```python
from build123d import *

# Parameters (mm, degrees)
SKETCH1_W                      = 40.11
SKETCH1_H                      = 20
BOSS_EXTRUDE1_DEPTH            = 12
SKETCH2_W                      = 35
SKETCH2_H                      = 17
BOSS_EXTRUDE2_DEPTH            = 6
SHELL1_START                   = 3.155
SHELL1_DEPTH                   = 33.8
SHELL1_START_2                 = 0.6
SHELL1_2_OUTLINE_W             = 18.8
SHELL1_2_OUTLINE_H             = 22.8
SHELL1_2_DEPTH                 = 38.91
SHELL1_START_3                 = -3.9
SHELL1_3_OUTLINE_R             = 0.1
SHELL1_3_DEPTH                 = 4.5
CUT_EXTRUDE1_REACH             = 48.398
SKETCH4_W                      = 30.63
SKETCH4_H                      = 5.52
CUT_EXTRUDE1_DIRECTION_2_REACH = 48.398
BOSS_EXTRUDE3_START            = 9.13
SKETCH5_W                      = 10.98
SKETCH5_H                      = 24.92
BOSS_EXTRUDE3_DEPTH            = 1.74
FILLET1_R                      = 2


# Read off the part's stored shape, not the designer's step: Shell1
with BuildPart() as part:
    # Sketch1 → Boss-Extrude1 (new, symmetric)
    with BuildSketch(Plane.XY):
        with Locations((20.055, 10)):
            Rectangle(SKETCH1_W, SKETCH1_H)
    extrude(amount=BOSS_EXTRUDE1_DEPTH, both=True)

    # Sketch2 → Boss-Extrude2 (add, symmetric)
    with BuildSketch(Plane.XY):
        with Locations((20.055, -8.5)):
            Rectangle(SKETCH2_W, SKETCH2_H)
    extrude(amount=BOSS_EXTRUDE2_DEPTH, both=True)

    # Sketch3 → Revolve1 (revolve)
    with BuildSketch(Plane.XY, mode=Mode.PRIVATE) as revolve1_sk:
        with BuildLine():
            Line((0, 0), (-3.5, 0))
            Line((-3.5, 0), (-3.5, -0.45))
            Line((-3.5, -0.45), (-4, -0.45))
            ThreePointArc((-4, -0.45), (-4.353553391, -0.303553391), (-4.5, 0.05))
            Line((-4.5, 0.05), (-4.5, 0.7))
            Line((-4.5, 0.7), (0, 0.7))
            Line((0, 0.7), (0, 0))
        make_face()
    revolve(revolve1_sk.sketch.rotate(Axis((0, 0.7, 0), (-1, 0, 0)), 180), axis=Axis((0, 0.7, 0), (-1, 0, 0)))

    # Shell1 outline → Shell1 (cut)
    with BuildSketch(Plane.YZ.offset(SHELL1_START)):
        Polygon((0.6, -5.4), (0.6, -11.4), (19.4, -11.4), (19.4, 11.4), (0.6, 11.4), (0.6, 5.4), (-17, 5.4), (-17, -5.4), align=None)
    extrude(amount=SHELL1_DEPTH, mode=Mode.SUBTRACT)

    # Shell1 2 outline → Shell1 2 (cut)
    with BuildSketch(Plane.YZ.offset(SHELL1_START_2)):
        with Locations((10, 0)):
            Rectangle(SHELL1_2_OUTLINE_W, SHELL1_2_OUTLINE_H)
    extrude(amount=SHELL1_2_DEPTH, mode=Mode.SUBTRACT)

    # Shell1 3 outline → Shell1 3 (cut)
    with BuildSketch(Plane.YZ.offset(SHELL1_START_3)):
        with Locations((0.7, 0)):
            Circle(SHELL1_3_OUTLINE_R)
    extrude(amount=SHELL1_3_DEPTH, mode=Mode.SUBTRACT)

    # Sketch4 → Cut-Extrude1 (cut, up to next)
    with BuildSketch(Plane.XY, mode=Mode.PRIVATE) as cut_extrude1_sk1:
        with Locations((20.055, -2.76)):
            Rectangle(SKETCH4_W, SKETCH4_H)
    cut_extrude1_tool1 = extrude(cut_extrude1_sk1.sketch, amount=-CUT_EXTRUDE1_REACH, mode=Mode.PRIVATE) & part.part
    add(cut_extrude1_tool1.solids().sort_by_distance((20.055, -2.76, 0))[0], mode=Mode.SUBTRACT)

    # Sketch4 → Cut-Extrude1 direction 2 (cut, up to next)
    with BuildSketch(Plane.XY, mode=Mode.PRIVATE) as cut_extrude1_direction_2_sk1:
        with Locations((20.055, -2.76)):
            Rectangle(SKETCH4_W, SKETCH4_H)
    cut_extrude1_direction_2_tool1 = extrude(cut_extrude1_direction_2_sk1.sketch, amount=CUT_EXTRUDE1_DIRECTION_2_REACH, mode=Mode.PRIVATE) & part.part
    add(cut_extrude1_direction_2_tool1.solids().sort_by_distance((20.055, -2.76, 0))[0], mode=Mode.SUBTRACT)

    # Sketch5 → Boss-Extrude3 (add)
    with BuildSketch(Plane.ZY.offset(-20.055).offset(BOSS_EXTRUDE3_START)):
        with Locations((0, 6.94)):
            Rectangle(SKETCH5_W, SKETCH5_H)
    boss_extrude3 = extrude(amount=BOSS_EXTRUDE3_DEPTH)

    # Mirror1: Boss-Extrude3 across plane
    add(boss_extrude3.mirror(Plane.ZY.offset(-20.055)))

    # Fillet1
    fillet1_edges = [part.edges().sort_by_distance(p)[0] for p in [
        (40.11, 10, 12),
        (20.055, 20, 12),
        (0, 10, 12),
        (20.055, 20, -12),
        (40.11, 10, -12),
        (0, 10, -12),
        (0, 20, 0),
        (40.11, 20, 0),
    ]]
    fillet(fillet1_edges, radius=FILLET1_R)


solid = part.part
```
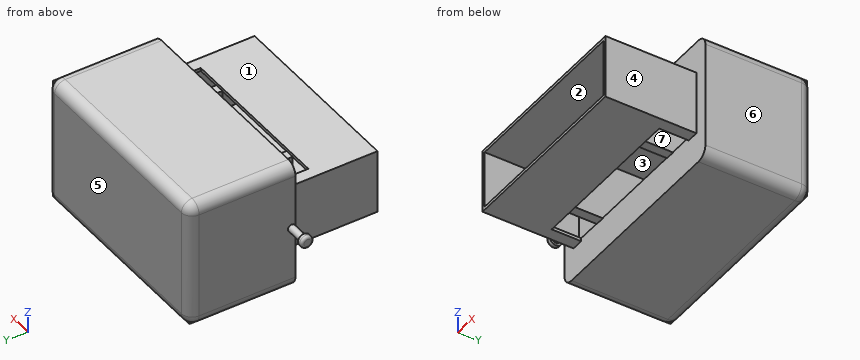
Geometry check sheet. Reference: the model listing, model coordinates, mm. Face numbers are marked on the shaded views. A direction names the side the tool comes from. Give positions to 0.01 mm unless a question says otherwise; leave off trailing zeros. Order: outer loops, then holes, each group sorted by start corner. A loop starts at its lowest first (then second) coordinate and runs counter-clockwise, first axis right, second up. Notation, with made-up numbers: (-14.5, 1.25) - (6.5, 1.25) arc R20 cw to (6.5, 38.25) - close; hole circle Ø4 at (70, 77.5). An arc over 180 degrees is marked (long way). Answer in a Markdown table with one row per item. Add a question column.
Q1. Gauge pin test, flat ends, axial feed: pin 1 (0.5 mm diameter, centred on x = 30, y = -2.5, fed in from -Z); pin 2 (4 mm diameter, centred on x = 8, y = -5, fed in from +Z); pin 3 (5 mm diameter, centred on x = 11, y = -12.5, fed in from -Z). Record the tip position at first contact, or that the pin passes through.
Q2. Cross-section at C-C, the plane z = 7.75. Enter the section's corners in (x, y).
Q3. Material ranges on probe 1 along X at (y, z) = (3.5, 2.5) (3 decimals); probe 2 along X at (y, z) = (-1, 1) (3 decimals); probe 3 along Z at (x, y) = (-1.6, 0.7), recorded low to high. Write a range as from..to.
Q4. Cross-section at A-A, the plane y = 3. Enter the section's corners in (x, z) (3 decimals).
Q5. Mould release check, pull along X, two halves, no side actions. Record for the marked faces 5, 6 and 7: pulls with the +X half, pulls with the -X half, needs draft (parallel to the pull), parting line crosses it, or undercut.
Q6. Cross-section at B-B, the plane x = 32.5. Enter the section's corners in (y, z), then the cut area to 3 significant figures.
Q7. Tool access check on the marked faces 1, 2, 3 and 4. Record the directions out of +Z, -Z, +X, -X, +Y, -Y that give a thin tool (end or side, any length) a straight path to the whole face; none if there is none.
Q8. Cross-section at D-D, the plane z = 4. Enter the section's corners in (x, y) (3 decimals), then the cut area to 3 significant figures.
Check values:
| question | item | result |
|---|---|---|
| 1 | pin 1 | stops at z = -5.49 |
| 1 | pin 2 | stops at z = 6 |
| 1 | pin 3 | stops at z = -6 |
| 2 | outline | (0, 0) - (40.11, 0) - (40.11, 18) arc R2 ccw to (38.11, 20) - (2, 20) arc R2 ccw to (0, 18) - close; hole (0.6, 0.6) - (39.51, 0.6) - (39.51, 19.4) - (0.6, 19.4) - close |
| 3 | probe 1 | x = 0..0.6, 9.185..10.925, 29.185..30.925, 39.51..40.11 |
| 3 | probe 2 | x = 2.555..3.155, 9.185..10.925, 29.185..30.925, 36.955..37.555 |
| 3 | probe 3 | z = -0.7..-0.1, 0.1..0.7 |
| 4 | outline | (0, -10) arc R2 ccw to (2, -12) - (38.11, -12) arc R2 ccw to (40.11, -10) - (40.11, 10) arc R2 ccw to (38.11, 12) - (2, 12) arc R2 ccw to (0, 10) - close; (9.185, -5.49) - (10.925, -5.49) - (10.925, 5.49) - (9.185, 5.49) - close; (29.185, -5.49) - (30.925, -5.49) - (30.925, 5.49) - (29.185, 5.49) - close; hole (0.6, -11.4) - (39.51, -11.4) - (39.51, 11.4) - (0.6, 11.4) - close |
| 5 | face 5 | needs draft |
| 5 | face 6 | pulls with the +X half |
| 5 | face 7 | undercut |
| 6 | outline | (-17, -6) - (-5.52, -6) - (-5.52, -5.4) - (-17, -5.4) - close; (-17, 5.4) - (-5.52, 5.4) - (-5.52, 6) - (-17, 6) - close; (0, -12) - (18, -12) arc R2 ccw to (20, -10) - (20, 10) arc R2 ccw to (18, 12) - (0, 12) - (0, 5.4) - (0.6, 5.4) - (0.6, 11.4) - (19.4, 11.4) - (19.4, -11.4) - (0.6, -11.4) - (0.6, -5.4) - (0, -5.4) - close |
| 6 | area | 56.9 mm^2 |
| 7 | face 1 | +Z, +X, -X, -Y |
| 7 | face 2 | -Y |
| 7 | face 3 | none |
| 7 | face 4 | +Z, -Z, +X, -Y |
| 8 | outline | (0, 0) - (2.555, 0) - (2.555, -17) - (3.155, -17) - (3.155, 0.6) - (0.6, 0.6) - (0.6, 19.4) - (9.185, 19.4) - (9.185, -5.52) - (10.925, -5.52) - (10.925, 19.4) - (29.185, 19.4) - (29.185, -5.52) - (30.925, -5.52) - (30.925, 19.4) - (39.51, 19.4) - (39.51, 0.6) - (36.955, 0.6) - (36.955, -17) - (37.555, -17) - (37.555, 0) - (40.11, 0) - (40.11, 18) arc R2 ccw to (38.11, 20) - (2, 20) arc R2 ccw to (0, 18) - close |
| 8 | area | 156 mm^2 |
